```python
from build123d import *

# Parameters (mm, degrees)
F0_W     = 128
F0_H     = 26
F1_DEPTH = 4
F3_DEPTH = 15
F4_W     = 128
F4_H     = 26
F5_DEPTH = 4


# Not quite as in the source:
# - a feature names something its author has since deleted; it is built from what else it names


with BuildPart() as f1:
    # F0 (on Top) → F1 (new body)
    with BuildSketch(Plane.XY):
        with Locations((-64, -13)):
            Rectangle(F0_W, F0_H)
    extrude(amount=F1_DEPTH)

    # F2 (on face) → F3 (join)
    with BuildSketch(Plane.XY.offset(4)):
        Polygon((-88.4999999069, 0), (-103.4999999069, 0), (-103.4999999069, -14.9287388836), (-118.4999999069, -14.9287388836), (-118.4999999069, 0), (-128, 0), (-128, -26), (0, -26), (0, 0), (-13.5, 0), (-13.5, -15.0637076219), (-28.5, -15.0637076219), (-28.5, 0), (-43.4999999069, 0), (-43.4999999069, -15), (-58.4999999069, -15), (-58.4999999069, 0), (-73.4999999069, 0), (-73.4999999069, -15.0510713975), (-88.4999999069, -15.0510713975), align=None)
    extrude(amount=F3_DEPTH)

    # F4 (on face) → F5 (join)
    with BuildSketch(Plane.XY.offset(19)):
        with Locations((-64, -13)):
            Rectangle(F4_W, F4_H)
    extrude(amount=F5_DEPTH)


solid = f1.part
```
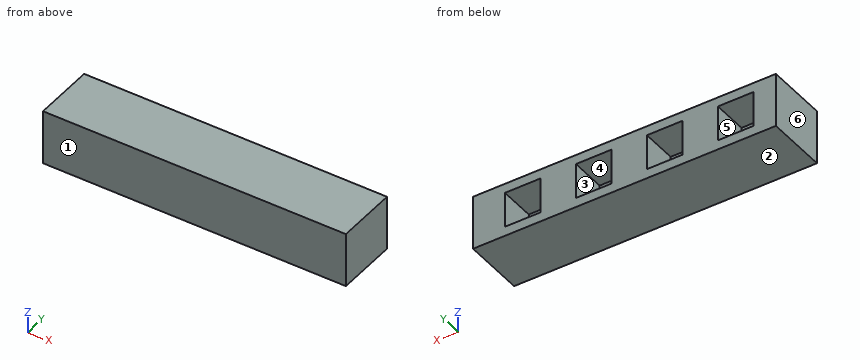
Work out the finished part from the listing and answer in its coordinate system (mm). Face numbers are marked on the shaded views. A direction names the side the tool comes from. Coordinates: 2 decimals unless noted, no trailing zeros. Write each loop counter-clockwise with the first axis right and the second up, starting at its lowest first coordinate (ties: lowest second). Pieces come first, ordered by that corner, then holes.
Q1. A cutting plane is placed at A-A, the plane x = -22. Give the vertices of the cut face in (y, z).
Q2. Which of the six approach directions +Z, -Z, +X, -X, +Y, -Y give full straight-line access (tool end or side, diameter ignored) to the marked faces 5 and 6?
Q3. Determine the mould class of the marked faces 1, 2, 3 and 4 for opening direction Z: released by +Z, released by -Z, zero draft, split by the parting line, or undercut.
Q4. A cutting plane is placed at D-D, the plane x = -51. Give the vertices of the cut face in (y, z), then the cut area to 3 significant figures.
Q5. A cutting plane is placed at B-B, the plane y = -9.75. Give the vertices of the cut face in (x, z).
Q6. A cutting plane is placed at C-C, the plane z = 17.75. Give the vertices of the cut face in (x, y).
Q7. Each of these flat-tipped pins is pushed along its axis until it touches: pin 1 Ø7.5 at (x, z) = (-54, 14) entering from +Y; pin 2 Ø4.5 at (x, z) = (-113, 8.5) entering from +Y. Where does it stop, or does it pass through?
Q8. Find the intervals of material crossed by line 1 (X direction, y = -8.25, z = 16.25); line 2 (Z direction, x = -51.5, y = -10.75); line 3 (Y direction, x = -81.5, z = 8.25), in increasing order.
Findings below:
1. outline: (-26, 0) - (0, 0) - (0, 4) - (-15.06, 4) - (-15.06, 19) - (0, 19) - (0, 23) - (-26, 23) - close
2. face 5: +Y
2. face 6: +Z, -Z, -X, +Y, -Y
3. face 1: zero draft
3. face 2: released by -Z
3. face 3: undercut
3. face 4: undercut
4. outline: (-26, 0) - (0, 0) - (0, 4) - (-15, 4) - (-15, 19) - (0, 19) - (0, 23) - (-26, 23) - close
4. area: 373 mm2
5. outline: (-128, 0) - (0, 0) - (0, 23) - (-128, 23) - close; hole (-118.5, 4) - (-103.5, 4) - (-103.5, 19) - (-118.5, 19) - close; hole (-88.5, 4) - (-73.5, 4) - (-73.5, 19) - (-88.5, 19) - close; hole (-58.5, 4) - (-43.5, 4) - (-43.5, 19) - (-58.5, 19) - close; hole (-28.5, 4) - (-13.5, 4) - (-13.5, 19) - (-28.5, 19) - close
6. outline: (-128, -26) - (0, -26) - (0, 0) - (-13.5, 0) - (-13.5, -15.06) - (-28.5, -15.06) - (-28.5, 0) - (-43.5, 0) - (-43.5, -15) - (-58.5, -15) - (-58.5, 0) - (-73.5, 0) - (-73.5, -15.05) - (-88.5, -15.05) - (-88.5, 0) - (-103.5, 0) - (-103.5, -14.93) - (-118.5, -14.93) - (-118.5, 0) - (-128, 0) - close
7. pin 1: stops at y = -15
7. pin 2: stops at y = -14.93
8. line 1: x = -128 to -118.5, -103.5 to -88.5, -73.5 to -58.5, -43.5 to -28.5, -13.5 to 0
8. line 2: z = 0 to 4, 19 to 23
8. line 3: y = -26 to -15.05
